```python
from build123d import *

# Parameters (mm, degrees)
SKETCH1_R           = 0.875
SKETCH1_R_2         = 3.5
BOSS_EXTRUDE1_DEPTH = 3
BOSS_EXTRUDE2_START = -2
SKETCH2_R           = 3.5
BOSS_EXTRUDE2_DEPTH = 2
FILLET1_R           = 3
FILLET2_R           = 0.3


with BuildPart() as part:
    # Sketch1 → Boss-Extrude1 (new body)
    with BuildSketch(Plane(origin=(0, 8.778505218, 0), x_dir=(1, 0, 0), z_dir=(0, 1, 0))):
        with BuildLine():
            Line((24.483909442, -36.009383283), (39.666515042, -34.709383283))
            ThreePointArc((39.666515042, -34.709383283), (43.483909442, -33.259383283), (47.301303841, -34.709383283))
            Line((47.301303841, -34.709383283), (60.330539136, -36.533530328))
            ThreePointArc((60.330539136, -36.533530328), (62.483909442, -39.009383283), (60.330539136, -41.485236238))
            Line((60.330539136, -41.485236238), (47.301303841, -43.309383283))
            ThreePointArc((47.301303841, -43.309383283), (43.483909442, -44.759383283), (39.666515042, -43.309383283))
            Line((39.666515042, -43.309383283), (24.483909442, -42.009383283))
            Line((24.483909442, -42.009383283), (24.483909442, -36.009383283))
        make_face()
        with Locations(Location((36.233909442, -39.009383283, 0), (0, 0, 270))):
            Circle(SKETCH1_R, mode=Mode.SUBTRACT)
        with Locations(Location((50.733909442, -39.009383283, 0), (0, 0, 270))):
            Circle(SKETCH1_R, mode=Mode.SUBTRACT)
        with Locations(Location((53.733909442, -39.009383283, 0), (0, 0, 270))):
            Circle(SKETCH1_R, mode=Mode.SUBTRACT)
        with Locations(Location((56.733909442, -39.009383283, 0), (0, 0, 270))):
            Circle(SKETCH1_R, mode=Mode.SUBTRACT)
        with Locations(Location((59.733909442, -39.009383283, 0), (0, 0, 270))):
            Circle(SKETCH1_R, mode=Mode.SUBTRACT)
        with Locations(Location((43.483909442, -39.009383283, 0), (0, 0, 270))):
            Circle(SKETCH1_R_2, mode=Mode.SUBTRACT)
        with BuildLine():
            Line((26.983909442, -37.509383283), (31.483909442, -37.509383283))
            ThreePointArc((31.483909442, -37.509383283), (32.983909442, -39.009383283), (31.483909442, -40.509383283))
            Line((31.483909442, -40.509383283), (26.983909442, -40.509383283))
            ThreePointArc((26.983909442, -40.509383283), (25.483909442, -39.009383283), (26.983909442, -37.509383283))
        make_face(mode=Mode.SUBTRACT)
    extrude(amount=BOSS_EXTRUDE1_DEPTH)

    # Sketch2 → Boss-Extrude2 (add)
    with BuildSketch(Plane(origin=(0, 11.778505218, 0), x_dir=(1, 0, 0), z_dir=(0, 1, 0)).offset(BOSS_EXTRUDE2_START)):
        with Locations(Location((43.483909442, -39.009383283, 0), (0, 0, 270))):
            Circle(SKETCH2_R)
    extrude(amount=BOSS_EXTRUDE2_DEPTH)

    # Fillet1
    fillet1_edges = [part.edges().sort_by_distance(p)[0] for p in [
        (24.483909442, 10.278505218, 42.009383283),
        (24.483909442, 10.278505218, 36.009383283),
    ]]
    fillet(fillet1_edges, radius=FILLET1_R)

    # Fillet2
    fillet2_edges = [part.edges().sort_by_distance(p)[0] for p in [
        (43.483909442, 11.778505218, 44.759383283),
        (53.815921489, 11.778505218, 42.39730976),
        (62.483909442, 11.778505218, 39.009383283),
        (53.815921489, 11.778505218, 35.621456805),
        (43.483909442, 11.778505218, 33.259383283),
        (33.447244034, 11.778505218, 42.776862547),
        (24.483909442, 11.778505218, 39.009383283),
        (33.447244034, 11.778505218, 35.241904019),
        (25.273953645, 11.778505218, 36.734671327),
        (25.273953645, 11.778505218, 41.284095239),
    ]]
    fillet(fillet2_edges, radius=FILLET2_R)


solid = part.part
```
Verification items for the finished model (mm, model axes). A direction names the side the tool comes from. Give positions to 0.01 mm unless a question says otherwise; leave off trailing zeros. Loops run counter-clockwise (first coordinate to the right, second up) from the corner with the lowest first, then second, coordinate; pieces in that order, holes last. Notation, with made-up numbers: M -40,36 L -4,36 A24 ccw -4,54 Z; hole C 36,28 d8. An arc over 180 degrees is marked long. One line per question, with ' | ' between items.
Item 1: Section check A-A, the plane y = 10.45. Record the cut outline in (x, z) (3 decimals), plus the area to 3 significant figures.
Completed:
outline: M 24.484,38.763 A3 ccw 27.228,35.774 L 39.667,34.709 A5.75 ccw 47.301,34.709 L 60.331,36.534 A2.5 ccw 60.331,41.485 L 47.301,43.309 A5.75 ccw 39.667,43.309 L 27.228,42.244 A3 ccw 24.484,39.255 Z; hole M 26.984,37.509 L 31.484,37.509 A1.5 ccw 31.484,40.509 L 26.984,40.509 A1.5 ccw Z; hole C 36.234,39.009 d1.75; hole C 50.734,39.009 d1.75; hole C 53.734,39.009 d1.75; hole C 56.734,39.009 d1.75; hole C 59.734,39.009 d1.75 | area: 252 mm^2
Item 2: Draft check along X on faces 1 (the face through (43.43, 10.11, 33.26)), 2 (the face through (33.59, 11.69, 35.32)), 3 (the face through (44, 9.779, 39)). Enter one of: +X half, -X half, draft (parallel to the pull), parting line (faces both ways), or undercut.
Completed:
face 1: parting line | face 2: -X half | face 3: undercut
Item 3: Tool access check on faces 4 (the face through (46.435, 9.272, 40.891)), 5 (the face through (53.67, 11.69, 42.33)), 6 (the face through (25.484, 10.258, 39.042)). Record the directions out of +Z, -Z, +X, -X, +Y, -Y that give a thin tool (end or side, any length) a straight path to the whole face; none if there is none.
Completed:
face 4: -Y | face 5: +Z, +X, +Y | face 6: +Y, -Y
Item 4: Depth check by flat-ended pin: P1, Ø3, axis at x = 46.5, z = 37.5, coming from the -Y side; P2, Ø1.6, axis at x = 59.73, z = 39.01, coming from the +Y side; P3, Ø1.5, axis at x = 50.5, y = 9.5, coming from the +Z side; P4, Ø0.9, axis at x = 30, y = 11, coming from the -Z side. Enter the tip coordinate at first touch or a pass-through.
Completed:
P1: stops at y = 8.78 | P2: passes through | P3: stops at z = 42.97 | P4: stops at z = 35.5
Item 5: Thickness scan on line 1 (Z direction, x = 28, y = 10.2); line 2 (Z direction, x = 53, y = 9.35); line 3 (X direction, y = 9.45, z = 41). Record the ranges inside material, lowest first. Write a range as [from, to].
Completed:
line 1: z = [35.71, 37.51], [40.51, 42.31] | line 2: z = [35.51, 38.53], [39.49, 42.51] | line 3: x = [25.04, 40.61], [46.36, 61.5]
